```python
from build123d import *

# Parameters (mm, degrees)
SKETCH1_W           = 17.78
SKETCH1_H           = 2.54
SKETCH1_R           = 0.5
BOSS_EXTRUDE1_DEPTH = 60
CUT_EXTRUDE1_START  = 8
CUT_EXTRUDE1_DEPTH  = 3
CUT_EXTRUDE2_START  = 28
CUT_EXTRUDE2_DEPTH  = 3
BOSS_EXTRUDE2_DEPTH = 35


with BuildPart() as part:
    # Sketch1 → Boss-Extrude1 (new body)
    with BuildSketch(Plane.XY):
        with BuildLine():
            Line((-5.200349399, -1.156583023), (-4.875189675, -1.110191708))
            ThreePointArc((-4.875189675, -1.110191708), (0.094891357, -4.999099482), (4.913809284, -0.924379964))
            Line((4.913809284, -0.924379964), (5.23403324, -0.993083178))
            ThreePointArc((5.23403324, -0.993083178), (0.083466761, -5.326758063), (-5.200349399, -1.156583023))
        make_face()
        with BuildLine():
            Line((-5.200349399, -1.156583023), (-8.89, -5.327411957))
            Line((-8.89, -5.327411957), (-9e-09, -5.327411957))
            ThreePointArc((-9e-09, -5.327411957), (-3.33314596, -4.155894148), (-5.200349399, -1.156583023))
        make_face()
        with Locations((0, -6.597411957)):
            Rectangle(SKETCH1_W, SKETCH1_H)
        with Locations((7.62, -6.597411957)):
            Circle(SKETCH1_R, mode=Mode.SUBTRACT)
        with Locations((5.08, -6.597411957)):
            Circle(SKETCH1_R, mode=Mode.SUBTRACT)
        with Locations((2.54, -6.597411957)):
            Circle(SKETCH1_R, mode=Mode.SUBTRACT)
        with Locations((0, -6.597411957)):
            Circle(SKETCH1_R, mode=Mode.SUBTRACT)
        with Locations((-2.54, -6.597411957)):
            Circle(SKETCH1_R, mode=Mode.SUBTRACT)
        with Locations((-5.08, -6.597411957)):
            Circle(SKETCH1_R, mode=Mode.SUBTRACT)
        with Locations((-7.62, -6.597411957)):
            Circle(SKETCH1_R, mode=Mode.SUBTRACT)
        with BuildLine():
            ThreePointArc((5.23403324, -0.993083178), (3.397848946, -4.103162281), (-9e-09, -5.327411957))
            Line((-9e-09, -5.327411957), (8.89, -5.327411957))
            Line((8.89, -5.327411957), (5.23403324, -0.993083178))
        make_face()
    extrude(amount=BOSS_EXTRUDE1_DEPTH)

    # Sketch2 → Cut-Extrude1 (cut, symmetric)
    with BuildSketch(Plane.XY.offset(CUT_EXTRUDE1_START)):
        with BuildLine():
            ThreePointArc((6.790005825, -2.837765364), (7.456750164, -4.429353345), (8.89, -5.390339932))
            Line((8.89, -5.390339932), (8.89, -6.424592971))
            ThreePointArc((8.89, -6.424592971), (6.41429556, -4.694977723), (5.853473578, -1.727460228))
            Line((5.853473578, -1.727460228), (6.790005825, -2.837765364))
        make_face()
    extrude(amount=CUT_EXTRUDE1_DEPTH, both=True, mode=Mode.SUBTRACT)

    # Sketch2<3> → Cut-Extrude2 (cut, symmetric)
    with BuildSketch(Plane.XY.offset(CUT_EXTRUDE2_START)):
        with BuildLine():
            ThreePointArc((6.790005825, -2.837765364), (7.456750164, -4.429353345), (8.89, -5.390339932))
            Line((8.89, -5.390339932), (8.89, -6.424592971))
            ThreePointArc((8.89, -6.424592971), (6.41429556, -4.694977723), (5.853473578, -1.727460228))
            Line((5.853473578, -1.727460228), (6.790005825, -2.837765364))
        make_face()
    extrude(amount=CUT_EXTRUDE2_DEPTH, both=True, mode=Mode.SUBTRACT)

    # Sketch2<4> → Boss-Extrude2 (add)
    with BuildSketch(Plane.XY):
        with BuildLine():
            Line((7.852011126, -3.078294754), (6.790005825, -2.837765364))
            ThreePointArc((6.790005825, -2.837765364), (7.456750164, -4.429353345), (8.89, -5.390339932))
            Line((8.89, -5.390339932), (9.432365549, -4.494075888))
            ThreePointArc((9.432365549, -4.494075888), (8.438966293, -4.01303031), (7.852011126, -3.078294754))
        make_face()
    extrude(amount=BOSS_EXTRUDE2_DEPTH)


solid = part.part
```
Part model, mm, in its own coordinate system. A direction names the side the tool comes from. Give positions to 0.01 mm unless a question says otherwise; leave off trailing zeros. Write each loop counter-clockwise with the first axis right and the second up, starting at its lowest first coordinate (ties: lowest second). Pieces come first, ordered by that corner, then holes. Notation, with made-up numbers: (24.25, 74.25) -> (73.25, 74.25) arc R23 cw to (73.25, 94.25) -> close; hole circle Ø9 at (50.25, -33). An arc over 180 degrees is marked (long way). Put each result on its own line as item: value. Start each with the question number.
Item 1: Pin check, flat tips, straight feed: pin 1 Ø3 at (y, z) = (-7, 37.5) entering from +X; pin 2 Ø4 at (y, z) = (-3, 27.5) entering from +X. Stop position of each tip, or through.
Item 2: Which spindle directions (+Z, -Z, +X, -X, +Y, -Y) get a long thin tool onto all of the face, cutting with end or side? Do faces 1 (the face through (6.68, -2.71, 36.25)), 2 (the face through (8.89, -7, 30)), 3 (the face through (7.1, -4.4, 11)). Say none if no direction does.
Item 3: Cut at C-C (z = 32.5). List the corners of the cut face in (x, y).
Item 4: Cut at B-B (z = 42). List the corners of the cut face in (x, y).
Item 5: Cut at D-D (x = -3.75). List the corners of the cut face in (y, z), then the cut area to 3 significant figures.
Item 6: Wall check: L1, parallel to Z at x = 6.5, y = -3.75; L2, parallel to Y at x = 0, z = 18; L3, parallel to X at y = -5.5, z = 34. Give the ranges that are in metal, low to high. Write a range as [from, to].
Item 7: Cut at A-A (y = -3.75). List the corners of the cut face in (x, z), then the cut area to 3 significant figures.
Item 8: Pull direction X, two halves, no side cores. Call faces 4 (the face through (7.1, -4.4, 5)), 5 (the face through (8, -4, 35)), 6 (the face through (-7.019, -3.213, 29.58)): pulls with the +X half, pulls with the -X half, needs draft (parallel to the pull), parting line crosses it, or undercut.
Answer list:
1. pin 1: stops at x = 8.89
1. pin 2: stops at x = 9.43
2. face 1: +Z, +X, +Y
2. face 2: +Z, -Z, +X, -Y
2. face 3: none
3. outline: (-8.89, -7.87) -> (8.89, -7.87) -> (8.89, -5.39) -> (9.43, -4.49) arc R2 cw to (7.85, -3.08) -> (6.79, -2.84) -> (5.23, -0.99) -> (4.91, -0.92) arc R5 cw to (-4.88, -1.11) -> (-5.2, -1.16) -> (-8.89, -5.33) -> close; hole circle Ø1 at (-7.62, -6.6); hole circle Ø1 at (-5.08, -6.6); hole circle Ø1 at (-2.54, -6.6); hole circle Ø1 at (0, -6.6); hole circle Ø1 at (2.54, -6.6); hole circle Ø1 at (5.08, -6.6); hole circle Ø1 at (7.62, -6.6)
4. outline: (-8.89, -7.87) -> (8.89, -7.87) -> (8.89, -5.33) -> (5.23, -0.99) -> (4.91, -0.92) arc R5 cw to (-4.88, -1.11) -> (-5.2, -1.16) -> (-8.89, -5.33) -> close; hole circle Ø1 at (-7.62, -6.6); hole circle Ø1 at (-5.08, -6.6); hole circle Ø1 at (-2.54, -6.6); hole circle Ø1 at (0, -6.6); hole circle Ø1 at (2.54, -6.6); hole circle Ø1 at (5.08, -6.6); hole circle Ø1 at (7.62, -6.6)
5. outline: (-7.87, 0) -> (-3.31, 0) -> (-3.31, 60) -> (-7.87, 60) -> close
5. area: 274 mm2
6. L1: z = [0, 5], [11, 25], [31, 60]
6. L2: y = [-7.87, -7.1], [-6.1, -5]
6. L3: x = [-8.89, 8.89]
7. outline: (-7.49, 0) -> (-3.31, 0) -> (-3.31, 60) -> (-7.49, 60) -> close; (3.31, 0) -> (8.19, 0) -> (8.19, 35) -> (7.56, 35) -> (7.56, 60) -> (3.31, 60) -> close; hole (5.97, 5) -> (7.04, 5) -> (7.04, 11) -> (5.97, 11) -> close; hole (5.97, 25) -> (7.04, 25) -> (7.04, 31) -> (5.97, 31) -> close
7. area: 516 mm2
8. face 4: undercut
8. face 5: needs draft
8. face 6: pulls with the -X half
